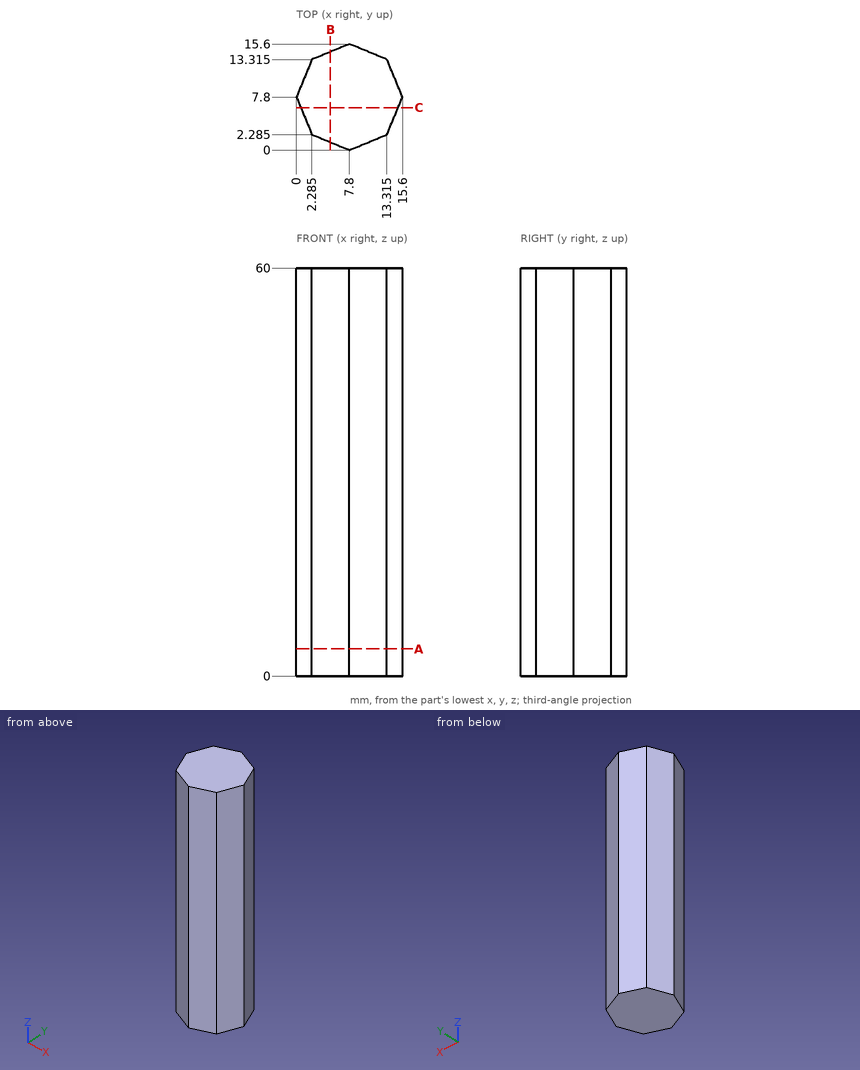
Here's the drawing with two shaded views (mm, measured from the low corner). I have some questions. Round coordinates to 2 decimals unless told otherwise and drop trailing zeros. Order: outer loops, then holes, each group sorted by start corner. A loop starts at its lowest first (then second) coordinate and runs counter-clockwise, first axis right, second up. Notation, with made-up numbers: M 78,19 L 103,19 A17 cw 103,37 Z; hole C -25.5,-18 d5. An arc over 180 degrees is marked long. Answer in a Markdown table with one row per item.
Item 1: Imagine slicing it at C-C, the plane y = 6.25. Write out the boundary of the cut face in (x, z).
A:
| item | result |
|---|---|
| outline | M 0.64,0 L 14.96,0 L 14.96,60 L 0.64,60 Z |
Item 2: Imagine slicing it at B-B, the plane x = 5. Write out the boundary of the cut face in (y, z).
A:
| item | result |
|---|---|
| outline | M 1.16,0 L 14.44,0 L 14.44,60 L 1.16,60 Z |
Item 3: If I drill on L1, parallel to X at y = 1, z = 49.5 (1 decimal); L2, parallel to X at y = 8.25, z = 48 (1 decimal); L3, parallel to Y at x = 7.25, z = 37, over which ranges is the centre line in solid material (lowest first)? Write a range as from..to.
A:
| item | result |
|---|---|
| L1 | x = 5.4..10.2 |
| L2 | x = 0.2..15.4 |
| L3 | y = 0.23..15.37 |
Item 4: Imagine slicing it at A-A, the plane z = 4. Write out the boundary of the cut face in (x, y) (1 decimal).
A:
| item | result |
|---|---|
| outline | M 0,7.8 L 2.3,2.3 L 7.8,0 L 13.3,2.3 L 15.6,7.8 L 13.3,13.3 L 7.8,15.6 L 2.3,13.3 Z |
Item 5: I'm going to push flat-ended pins straight in: pin 1 (2 mm diameter, centred on x = 11.5, z = 20.5, fed in from +Y); pin 2 (3 mm diameter, centred on x = 12.5, z = 11, fed in from -Y) (1 decimal); pin 3 (6 mm diameter, centred on y = 2, z = 52.5, fed in from +X). Where does each tip first touch, or does it pass through?
A:
| item | result |
|---|---|
| pin 1 | stops at y = 14.48 |
| pin 2 | stops at y = 1.3 |
| pin 3 | stops at x = 14.44 |
